The model under review builds one solid part; all positions refer to its coordinate system, in mm. Face numbers are marked on the shaded views. A direction names the side the tool comes from. Round coordinates to 2 decimals unless told otherwise and drop trailing zeros. Order: outer loops, then holes, each group sorted by start corner. A loop starts at its lowest first (then second) coordinate and runs counter-clockwise, first axis right, second up. Notation, with made-up numbers: M 45.25,38 L 65.25,38 A28 ccw 65.25,75 Z; hole C 78,52 d8. An arc over 180 degrees is marked long. Answer as a JSON object with one key per item and string values. Group by question number.
1) Consider section C-C, the plane z = 62.5. Write out the cut boundary in (x, y), then the cut area to 3 significant figures.
2) To check wall thickness, follow line 1 (Z direction, x = 103, y = 37); line 2 (X direction, y = 58, z = 68.3); line 3 (X direction, y = 44.85, z = 41). State the ranges of each line that lie inside material, in increasing order.
3) Insertion check: pin 1 Ø1.1 at (x, z) = (103, 26.5) entering from +Y; pin 2 Ø15.5 at (x, z) = (97.5, 53.5) entering from -Y; pin 3 Ø5.5 at (x, z) = (104.5, 57.5) entering from +Y; pin 4 Ø10.5 at (x, z) = (103, 26) entering from +Y. Each pin has a flat end and moves straight along its axis. Give the tip position at first contact, or say it passes through.
4) For the marked faces 1, 2 and 3, list the 3-axis set-ups (+Z, -Z, +X, -X, +Y, -Y) from which the entire face can be reached by the end or side of a thin tool; tool diameter is ignored.
5) The part is to be moulded in two halves that separate along X. For the marked faces 4, 5 and 6, say which applies: +X half, -X half, draft (parallel to the pull), parting line (faces both ways), or undercut.
6) Consider section A-A, the plane z = 34. Write out the cut boundary in (x, y), then the cut area to 3 significant figures.
7) Consider section B-B, the plane y = 19. Write out the cut boundary in (x, z), then the cut area to 3 significant figures.
8) Consider section D-D, the plane z = 26. Write out the cut boundary in (x, y), then the cut area to 3 significant figures.
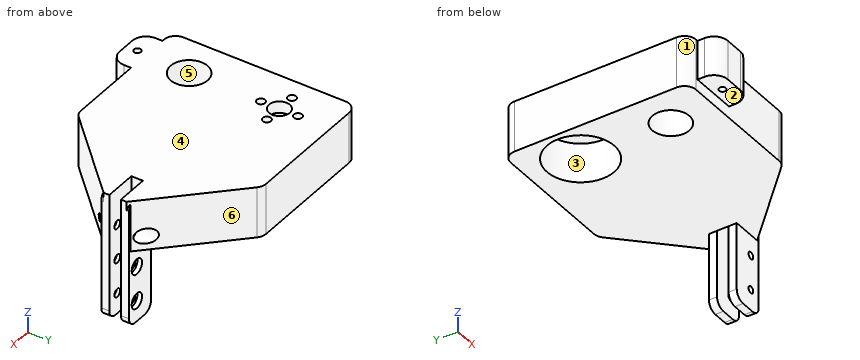
```python
from build123d import *

# Parameters (mm, degrees)
CYLINDER038_R       = 1.8
CYLINDER038_DEPTH   = 20
ARRAY001017_COUNT   = 4
CYLINDER031_R       = 4.5
CYLINDER031_DEPTH   = 6
CYLINDER030_R       = 16
CYLINDER030_DEPTH   = 5
CYLINDER032_R       = 14.5
CYLINDER032_DEPTH   = 30
CYLINDER033_R       = 1.8
CYLINDER033_DEPTH   = 8
CYLINDER035_R       = 1.5
CYLINDER035_DEPTH   = 10
CYLINDER034_R       = 3.3
CYLINDER034_DEPTH   = 20
ARRAY001002_Z_COUNT = 3
ARRAY001002_Z_PITCH = 15
BOX006_W            = 14
BOX006_H            = 5
BOX006_DEPTH        = 55
CYLINDER017_R       = 8
CYLINDER017_DEPTH   = 24
BOX005_W            = 14
BOX005_H            = 12
BOX005_DEPTH        = 55
FILLET006_R         = 4
CYLINDER039_R       = 1.5
CYLINDER039_DEPTH   = 30
BOX018_W            = 20
BOX018_H            = 10
BOX018_DEPTH        = 17
FILLET007_R         = 6
BOX004_W            = 95
BOX004_H            = 80
BOX004_DEPTH        = 22
CHAMFER_SIZE        = 35
FILLET005_R         = 5


with BuildPart() as lead_nut_attachment_bolt_hole_array:
    # Cylinder038 → Cylinder038 (new body)
    with BuildSketch(Plane(origin=(0, -8, -5), x_dir=(1, 0, 0), z_dir=(0, 0, 1))):
        Circle(CYLINDER038_R)
    extrude(amount=CYLINDER038_DEPTH)

    # Array001017: lead nut attachment bolt hole array ×4 about axis
    array001017_axis = Axis((0, 0, 0), (0, 0, 1))


with BuildPart() as lead_nut_attachment_bolt_hole_array_1:
    add(lead_nut_attachment_bolt_hole_array.part)
    for i in range(1, ARRAY001017_COUNT):
        add(lead_nut_attachment_bolt_hole_array.part.rotate(array001017_axis, i * 360 / ARRAY001017_COUNT))


with BuildPart() as hole_fusion001:
    # Cylinder031 → Cylinder031 (new body)
    with BuildSketch(Plane.XY):
        Circle(CYLINDER031_R)
    extrude(amount=CYLINDER031_DEPTH)

    # Fusion009: union lead nut attachment bolt hole array
    add(lead_nut_attachment_bolt_hole_array_1.part)


with BuildPart() as lean_nut_attachment_clone:
    # Cylinder030 → Cylinder030 (new body)
    with BuildSketch(Plane.XY):
        Circle(CYLINDER030_R)
    extrude(amount=CYLINDER030_DEPTH)

    # Cut005: cut hole fusion001
    add(hole_fusion001.part, mode=Mode.SUBTRACT)


with BuildPart() as lean_nut_attachment_clone_1:
    # Body001 placement: moved
    add(lean_nut_attachment_clone.part.moved(Location((17, 58, 17))))


with BuildPart() as backlash_nut_disk_hole:
    # Cylinder032 → Cylinder032 (new body)
    with BuildSketch(Plane(origin=(17, 58, -5), x_dir=(1, 0, 0), z_dir=(0, 0, 1))):
        Circle(CYLINDER032_R)
    extrude(amount=CYLINDER032_DEPTH)


with BuildPart() as attachment_hole001:
    # Cylinder033 → Cylinder033 (new body)
    with BuildSketch(Plane(origin=(0, 0, 0), x_dir=(1, 0, 0), z_dir=(0, 1, 0))):
        Circle(CYLINDER033_R)
    extrude(amount=CYLINDER033_DEPTH)


with BuildPart() as screwed_hole:
    # Cylinder035 → Cylinder035 (new body)
    with BuildSketch(Plane(origin=(0, -10, 0), x_dir=(1, 0, 0), z_dir=(0, 1, 0))):
        Circle(CYLINDER035_R)
    extrude(amount=CYLINDER035_DEPTH)


with BuildPart() as attachment_hole_array001:
    # Cylinder034 → Cylinder034 (new body)
    with BuildSketch(Plane(origin=(0, 8, 0), x_dir=(1, 0, 0), z_dir=(0, 1, 0))):
        Circle(CYLINDER034_R)
    extrude(amount=CYLINDER034_DEPTH)

    # Fusion013: union attachment hole001, screwed hole
    add(attachment_hole001.part)
    add(screwed_hole.part)

    # Array001002 Z: attachment hole array001 ×3


with BuildPart() as attachment_hole_array001_1:
    add(attachment_hole_array001.part)
    with Locations(*[(0, 0, i * ARRAY001002_Z_PITCH) for i in range(1, ARRAY001002_Z_COUNT)]):
        add(attachment_hole_array001.part)


with BuildPart() as attachment_hole_array001_2:
    # Array001002 placement: moved
    add(attachment_hole_array001_1.part.moved(Location((90, 36, -24))))


with BuildPart() as top_attachment_connector_extract:
    # Box006 → Box006 (new body)
    with BuildSketch(Plane(origin=(81, 37.5, -33), x_dir=(1, 0, 0), z_dir=(0, 0, 1))):
        with Locations((7, 2.5)):
            Rectangle(BOX006_W, BOX006_H)
    extrude(amount=BOX006_DEPTH)


with BuildPart() as obj1:
    # Cylinder017 → Cylinder017 (new body)
    with BuildSketch(Plane(origin=(17, 19, 0), x_dir=(1, 0, 0), z_dir=(0, 0, 1))):
        Circle(CYLINDER017_R)
    extrude(amount=CYLINDER017_DEPTH)

    # Fusion010: union backlash nut disk hole, attachment hole array001, top_attachment_connector_extract
    add(backlash_nut_disk_hole.part)
    add(attachment_hole_array001_2.part)
    add(top_attachment_connector_extract.part)


with BuildPart() as top_attachment_connector_fillet:
    # Box005 → Box005 (new body)
    with BuildSketch(Plane(origin=(81, 34, -33), x_dir=(1, 0, 0), z_dir=(0, 0, 1))):
        with Locations((7, 6)):
            Rectangle(BOX005_W, BOX005_H)
    extrude(amount=BOX005_DEPTH)

    # Fillet006
    fillet006_edges = [top_attachment_connector_fillet.edges().sort_by_distance(p)[0] for p in [
        (81, 40, 22),
        (81, 40, -33),
        (95, 40, 22),
        (95, 40, -33),
    ]]
    fillet(fillet006_edges, radius=FILLET006_R)


with BuildPart() as obj2:
    # Cylinder039 → Cylinder039 (new body)
    with BuildSketch(Plane(origin=(10, 5, 0), x_dir=(1, 0, 0), z_dir=(0, 0, 1))):
        Circle(CYLINDER039_R)
    extrude(amount=CYLINDER039_DEPTH)


with BuildPart() as obj3:
    # Box018 → Box018 (new body)
    with BuildSketch(Plane.XY):
        with Locations((10, 5)):
            Rectangle(BOX018_W, BOX018_H)
    extrude(amount=BOX018_DEPTH)

    # Fillet007
    fillet007_edges = [obj3.edges().sort_by_distance(p)[0] for p in [
        (0, 0, 8.5),
        (20, 0, 8.5),
    ]]
    fillet(fillet007_edges, radius=FILLET007_R)

    # Cut014: cut obj2
    add(obj2.part, mode=Mode.SUBTRACT)


with BuildPart() as obj3_1:
    # Cut014 placement: moved
    add(obj3.part.moved(Location((6, -9, 5))))


with BuildPart() as obj4:
    # Box004 → Box004 (new body)
    with BuildSketch(Plane.XY):
        with Locations((47.5, 40)):
            Rectangle(BOX004_W, BOX004_H)
    extrude(amount=BOX004_DEPTH)

    # Chamfer
    chamfer_edges = [obj4.edges().sort_by_distance(p)[0] for p in [
        (95, 0, 11),
        (95, 80, 11),
    ]]
    chamfer(chamfer_edges, length=CHAMFER_SIZE)

    # Fillet005
    fillet005_edges = [obj4.edges().sort_by_distance(p)[0] for p in [
        (60, 0, 11),
        (60, 80, 11),
        (0, 80, 11),
        (0, 0, 11),
    ]]
    fillet(fillet005_edges, radius=FILLET005_R)

    # Fusion012: union top attachment connector fillet, obj3
    add(top_attachment_connector_fillet.part)
    add(obj3_1.part)

    # Cut006: cut obj1
    add(obj1.part, mode=Mode.SUBTRACT)

    # Fusion011: union lean nut attachment clone
    add(lean_nut_attachment_clone_1.part)


with BuildPart() as obj4_1:
    # Fusion011 placement: moved
    add(obj4.part.moved(Location((13, 0, 50))))


solid = obj4_1.part
```
Results list:
{
 "1": {"outline": "M 13,5 A5 ccw 18,0 L 19,0 L 19,-3 A6 ccw 25,-9 L 33,-9 A6 ccw 39,-3 L 39,0 L 70.93,0 A5 ccw 74.46,1.46 L 107,34 L 108,34 L 108,37.5 L 94,37.5 L 94,42.5 L 108,42.5 L 108,46 L 107,46 L 74.46,78.54 A5 ccw 70.93,80 L 18,80 A5 ccw 13,75 Z; hole C 30,58 d29; hole C 30,19 d16; hole C 29,-4 d3", "area": "5,590 mm^2"},
 "2": {"line 1": "17 to 24.2, 27.8 to 39.2, 42.8 to 54.2, 57.8 to 72", "line 2": "13 to 20.2, 23.8 to 25.5, 34.5 to 36.2, 39.8 to 95", "line 3": "94 to 99.7, 106.3 to 108"},
 "3": {"pin 1": "through", "pin 2": "y = 16.75", "pin 3": "y = 50.63", "pin 4": "y = 46"},
 "4": {"face 1": "+Z, -Z, -X, -Y", "face 2": "-Z, +X, -X, -Y", "face 3": "-Z"},
 "5": {"face 4": "draft", "face 5": "undercut", "face 6": "+X half"},
 "6": {"outline": "M 94,34 L 108,34 L 108,37.5 L 94,37.5 Z; M 94,42.5 L 108,42.5 L 108,46 L 94,46 Z", "area": "98.0 mm^2"},
 "7": {"outline": "M 13,50 L 22,50 L 22,72 L 13,72 Z; M 38,50 L 92,50 L 92,72 L 38,72 Z", "area": "1,390 mm^2"},
 "8": {"outline": "M 94,34 L 101.5,34 L 101.5,36 L 101.2,36 L 101.2,37.5 L 94,37.5 Z; M 94,42.5 L 101.2,42.5 L 101.2,44 L 99.7,44 L 99.7,46 L 94,46 Z; M 104.5,34 L 108,34 L 108,37.5 L 104.8,37.5 L 104.8,36 L 104.5,36 Z; M 104.8,42.5 L 108,42.5 L 108,46 L 106.3,46 L 106.3,44 L 104.8,44 Z", "area": "68.0 mm^2"}
}
